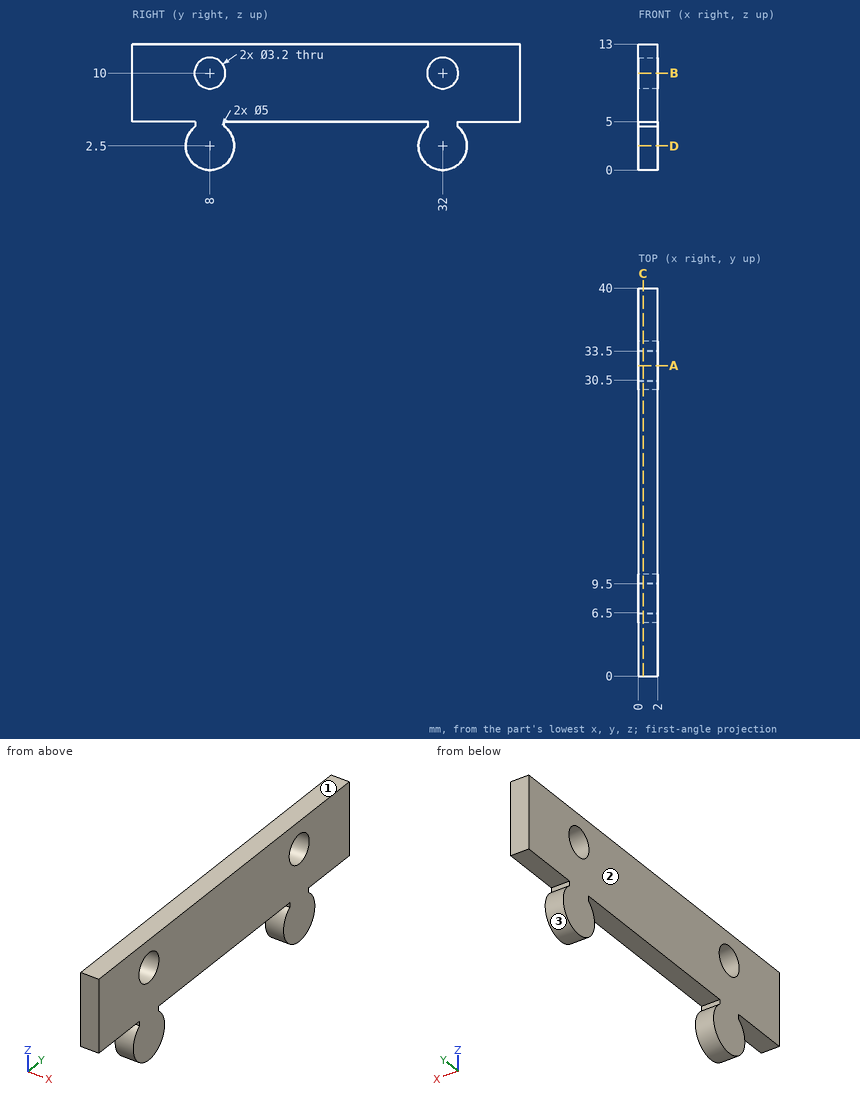
Source: three-view drawing plus pictorial views. Frame: mm from the lowest corner of the part. Round coordinates to 2 decimals unless told otherwise and drop trailing zeros. Loops run counter-clockwise (first coordinate to the right, second up) from the corner with the lowest first, then second, coordinate; pieces in that order, holes last.
1. Section query D-D on z = 2.5. Output: boundary loops of the cut face in (x, y), and give its area (3 significant figures).
2. Contact query for flat-ended pins moving along their axis: pin 1 (1 mm diameter, centred on x = 1.5, z = 2.5, fed in from -Y); pin 2 (0.6 mm diameter, centred on x = 1.5, z = 4.5, fed in from -Y); pin 3 (0.6 mm diameter, centred on x = 0.5, y = 3, fed in from -Z). Output: stop coordinate, or through.
3. Ray query, L1, parallel to Y at x = 0.9, z = 10; L2, parallel to Y at x = 1.55, z = 2.5; L3, parallel to Y at x = 0.8, z = 11. Return the intervals inside material, ascending.
4. Section query B-B on z = 10. Output: boundary loops of the cut face in (x, y), and give its area (3 significant figures).
5. Section query A-A on y = 32. Output: boundary loops of the cut face in (x, z), and give its area (3 significant figures).
6. Mould query, pull axis Z, two halves, no side actions, for the marked faces 1, 2 and 3. Classes: released by +Z, released by -Z, zero draft, split by the parting line, or undercut.
7. Section query C-C on x = 0.5. Output: boundary loops of the cut face in (y, z), and give its area (3 significant figures).
Answers below:
1. outline: (0, 5.5) - (2, 5.5) - (2, 10.5) - (0, 10.5) - close; (0, 29.5) - (2, 29.5) - (2, 34.5) - (0, 34.5) - close
1. area: 20.0 mm2
2. pin 1: stops at y = 5.5
2. pin 2: stops at y = 6.17
2. pin 3: stops at z = 5
3. L1: y = 0 to 6.4, 9.6 to 30.4, 33.6 to 40
3. L2: y = 5.5 to 10.5, 29.5 to 34.5
3. L3: y = 0 to 6.75, 9.25 to 30.75, 33.25 to 40
4. outline: (0, 0) - (2, 0) - (2, 6.4) - (0, 6.4) - close; (0, 9.6) - (2, 9.6) - (2, 30.4) - (0, 30.4) - close; (0, 33.6) - (2, 33.6) - (2, 40) - (0, 40) - close
4. area: 67.2 mm2
5. outline: (0, 0) - (2, 0) - (2, 8.4) - (0, 8.4) - close; (0, 11.6) - (2, 11.6) - (2, 13) - (0, 13) - close
5. area: 19.6 mm2
6. face 1: released by +Z
6. face 2: zero draft
6. face 3: undercut
7. outline: (0, 5) - (6.5, 5) - (6.5, 4.5) arc R2.5 ccw (long way) to (9.5, 4.5) - (9.5, 5) - (30.5, 5) - (30.5, 4.5) arc R2.5 ccw (long way) to (33.5, 4.5) - (33.5, 5) - (40, 5) - (40, 13) - (0, 13) - close; hole circle Ø3.2 at (8, 10); hole circle Ø3.2 at (32, 10)
7. area: 344 mm2
